Source: three-view drawing plus pictorial views. Frame: mm from the lowest corner of the part. A direction names the side the tool comes from. Round coordinates to 2 decimals unless told otherwise and drop trailing zeros. Return JSON: item names as keys, results as strings. Group by question number.
1) Material intervals for line 1 (X direction, y = 13.75, z = 4.5); line 2 (X direction, y = 4.5, z = 11.5); line 3 (Y direction, x = 11.25, z = 5.75), sorted ascending. Write a range as from..to.
2) Contact query for flat-ended pins moving along their axis: P1, Ø5, axis at x = 3, z = 5.5, coming from the +Y side; P2, Ø1, axis at y = 4.5, z = 9, coming from the +X side. Output: stop coordinate, or through.
3) Access query for the marked faces 1, 2 and 3. Directions: +Z, -Z, +X, -X, +Y, -Y. A direction counts if a zero-diameter tool reaches every point of the face in a straight line with its end or side. Return the directions, or none.
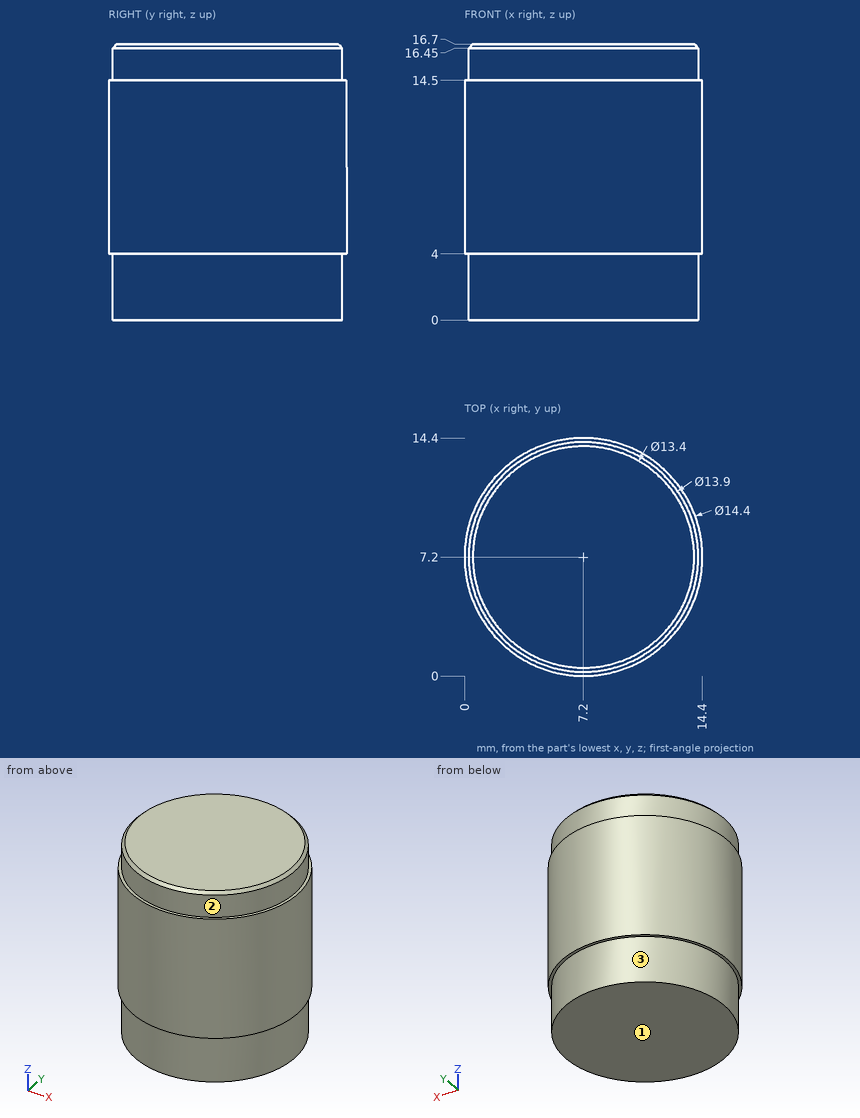
Returned:
{
 "1": {"line 1": "x = 4.21..10.19", "line 2": "x = 0.53..13.87", "line 3": "y = 1.25..13.15"},
 "2": {"P1": "stops at y = 14.2", "P2": "stops at x = 14.06"},
 "3": {"face 1": "-Z, +X, -X, +Y, -Y", "face 2": "+Z", "face 3": "-Z"}
}
